```python
from build123d import *

# Parameters (mm, degrees)
SKETCH_1_W          = 18
SKETCH_1_H          = 18
EXTRUDE_1_DEPTH     = 0.8
SKETCH_2_R          = 1.75
CUT_EXTRUDE_1_DEPTH = 26.468411808
SKETCH_3_R          = 4
EXTRUDE_2_DEPTH     = 2.5


with BuildPart() as part:
    # 草图1 → 凸台-拉伸1 (new body)
    with BuildSketch(Plane(origin=(0, 0, 0), x_dir=(1, 0, 0), z_dir=(0, 1, 0))):
        with Locations((9, 9)):
            Rectangle(SKETCH_1_W, SKETCH_1_H)
    extrude(amount=EXTRUDE_1_DEPTH)

    # 草图2 → 切除-拉伸1 (cut, through all)
    with BuildSketch(Plane(origin=(0, 0.8, 0), x_dir=(1, 0, 0), z_dir=(0, 1, 0))):
        with Locations(Location((3, 15, 0), (0, 0, 270))):
            Circle(SKETCH_2_R)
        with Locations(Location((15, 15, 0), (0, 0, 270))):
            Circle(SKETCH_2_R)
        with Locations(Location((15, 3, 0), (0, 0, 270))):
            Circle(SKETCH_2_R)
        with Locations(Location((3, 3, 0), (0, 0, 270))):
            Circle(SKETCH_2_R)
    extrude(amount=-CUT_EXTRUDE_1_DEPTH, mode=Mode.SUBTRACT)

    # 草图3 → 凸台-拉伸2 (add)
    with BuildSketch(Plane(origin=(0, 0.8, 0), x_dir=(1, 0, 0), z_dir=(0, 1, 0))):
        with Locations(Location((9, 9, 0), (0, 0, 90))):
            Circle(SKETCH_3_R)
    extrude(amount=EXTRUDE_2_DEPTH)


solid = part.part
```
The model under review builds one solid part; all positions refer to its coordinate system, in mm. A direction names the side the tool comes from. Round coordinates to 2 decimals unless told otherwise and drop trailing zeros. Order: outer loops, then holes, each group sorted by start corner. A loop starts at its lowest first (then second) coordinate and runs counter-clockwise, first axis right, second up.
Item 1: For pin 1 (3 mm diameter, centred on x = 13.5, z = -14.5, fed in from +Y), flat-tipped, find the tip position at first contact; note if it passes through.
Working result:
pin 1: stops at y = 0.8
Item 2: Add section B-B, the plane z = -15. State the section outline as (x, y) points, and give its area (3 significant figures).
Working result:
outline: (0, 0) - (1.25, 0) - (1.25, 0.8) - (0, 0.8) - close; (4.75, 0) - (13.25, 0) - (13.25, 0.8) - (4.75, 0.8) - close; (16.75, 0) - (18, 0) - (18, 0.8) - (16.75, 0.8) - close
area: 8.80 mm2
Item 3: Machinability: for faces 4 (the flat face through (9, 0, -9)), 5 (the flat face through (5, 0.8, -11)), which of the approach directions +Z, -Z, +X, -X, +Y, -Y give a long, thin tool a straight path to every point of the face, cutting with its end or side? Answer none if there is none.
Working result:
face 4: +Z, -Z, +X, -X, -Y
face 5: +Y
Item 4: Add section D-D, the plane z = -9. State the section outline as (x, y) points, and give its area (3 significant figures).
Working result:
outline: (0, 0) - (18, 0) - (18, 0.8) - (13, 0.8) - (13, 3.3) - (5, 3.3) - (5, 0.8) - (0, 0.8) - close
area: 34.4 mm2
Item 5: To check wall thickness, follow probe 1 along X at (y, z) = (0.2, -3); probe 2 along Z at (x, y) = (13.75, 0.7); probe 3 along X at (y, z) = (0.65, -4.5). State the ranges of each line that lie inside material, in increasing order.
Working result:
probe 1: x = 0 to 1.25, 4.75 to 13.25, 16.75 to 18
probe 2: z = -18 to -16.22, -13.78 to -4.22, -1.78 to 0
probe 3: x = 0 to 2.1, 3.9 to 14.1, 15.9 to 18
Item 6: Add section C-C, the plane y = 0.3. State the section outline as (x, z) points, and give its area (3 significant figures).
Working result:
outline: (0, -18) - (18, -18) - (18, 0) - (0, 0) - close; hole circle Ø3.5 at (3, -15); hole circle Ø3.5 at (3, -3); hole circle Ø3.5 at (15, -15); hole circle Ø3.5 at (15, -3)
area: 286 mm2
Item 7: Add section A-A, the plane x = 15. State the section outline as (y, z) points.
Working result:
outline: (0, -18) - (0.8, -18) - (0.8, -16.75) - (0, -16.75) - close; (0, -13.25) - (0.8, -13.25) - (0.8, -4.75) - (0, -4.75) - close; (0, -1.25) - (0.8, -1.25) - (0.8, 0) - (0, 0) - close
Item 8: Draft analysis for pull direction X (two halves, no side actions). For faces 1 (the cylindrical face through (11.4, 2, -5.8)), 2 (the flat face through (9, 3.3, -9)), 3 (the cylindrical face through (16.5, 0.4, -14.1)), state which applies: released by +X, released by -X, zero draft, split by the parting line, or undercut.
Working result:
face 1: split by the parting line
face 2: zero draft
face 3: undercut
